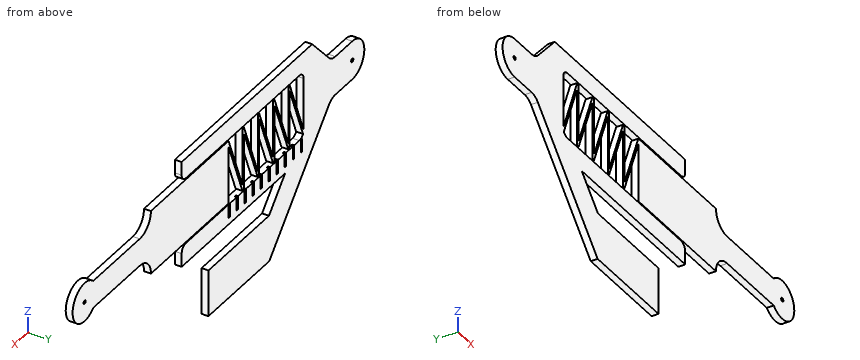
```python
from build123d import *

# Parameters (mm, degrees)
SKETCH3_R           = 0.8255
BOSS_EXTRUDE1_DEPTH = 3.175
SKETCH4_W           = 1
SKETCH4_H           = 6.35
CUT_EXTRUDE1_DEPTH  = 1


with BuildPart() as part:
    # Sketch3 → Boss-Extrude1 (new body)
    with BuildSketch(Plane(origin=(0, 0, 0), x_dir=(1, 0, 0), z_dir=(0, 1, 0))):
        with BuildLine():
            Line((-187.300108, 9), (-200.000108, 9))
            ThreePointArc((-200.000108, 9), (-209.000108, 0), (-200.000108, -9))
            Line((-200.000108, -9), (-187.300108, -9))
            ThreePointArc((-187.300108, -9), (-184.751148517, -9.534047322), (-182.630933912, -11.046360455))
            Line((-182.630933912, -11.046360455), (-170.000108, -24.75))
            Line((-170.000108, -24.75), (-72.500108, -24.75))
            Line((-72.500108, -24.75), (-72.500108, -18.525))
            ThreePointArc((-72.500108, -18.525), (-73.43004397, -16.27993597), (-75.675108, -15.35))
            Line((-75.675108, -15.35), (-160.475108, -15.35))
            ThreePointArc((-160.475108, -15.35), (-162.72017203, -14.42006403), (-163.650108, -12.175))
            Line((-163.650108, -12.175), (-163.650108, 12.175))
            Line((-163.650108, 12.175), (-153.250108, -14.85))
            Line((-153.250108, -14.85), (-152.250108, -14.85))
            Line((-152.250108, -14.85), (-152.250108, 12.090726648))
            Line((-152.250108, 12.090726648), (-141.820108, -14.732))
            Line((-141.820108, -14.732), (-140.820108, -14.732))
            Line((-140.820108, -14.732), (-140.820108, 12.090726648))
            Line((-140.820108, 12.090726648), (-130.390108, -14.732))
            Line((-130.390108, -14.732), (-129.390108, -14.732))
            Line((-129.390108, -14.732), (-129.390108, 12.090726648))
            Line((-129.390108, 12.090726648), (-118.960108, -14.732))
            Line((-118.960108, -14.732), (-117.960108, -14.732))
            Line((-117.960108, -14.732), (-117.960108, 12.090726648))
            Line((-117.960108, 12.090726648), (-107.530108, -14.732))
            Line((-107.530108, -14.732), (-49.530108, -14.732))
            ThreePointArc((-49.530108, -14.732), (-47.07507704, -8.80503096), (-41.148108, -6.35))
            Line((-41.148108, -6.35), (-6.377891501, -6.35))
            ThreePointArc((-6.377891501, -6.35), (9, 0), (-6.377891501, 6.35))
            Line((-6.377891501, 6.35), (-41.148108, 6.35))
            ThreePointArc((-41.148108, 6.35), (-47.07507704, 8.80503096), (-49.530108, 14.732))
            Line((-49.530108, 14.732), (-49.530108, 14.85))
            Line((-49.530108, 14.85), (-107.530108, 14.85))
            Line((-107.530108, 14.85), (-107.530108, -11.972726648))
            Line((-107.530108, -11.972726648), (-117.960108, 14.85))
            Line((-117.960108, 14.85), (-118.960108, 14.85))
            Line((-118.960108, 14.85), (-118.960108, -11.972726648))
            Line((-118.960108, -11.972726648), (-129.390108, 14.85))
            Line((-129.390108, 14.85), (-130.390108, 14.85))
            Line((-130.390108, 14.85), (-130.390108, -11.972726648))
            Line((-130.390108, -11.972726648), (-140.820108, 14.85))
            Line((-140.820108, 14.85), (-141.820108, 14.85))
            Line((-141.820108, 14.85), (-141.820108, -11.972726648))
            Line((-141.820108, -11.972726648), (-152.250108, 14.85))
            Line((-152.250108, 14.85), (-153.250108, 14.85))
            Line((-153.250108, 14.85), (-153.250108, -12.065668468))
            Line((-153.250108, -12.065668468), (-163.203485052, 13.798756035))
            ThreePointArc((-163.203485052, 13.798756035), (-162.044375279, 14.935077029), (-160.475108, 15.35))
            Line((-160.475108, 15.35), (-75.675108, 15.35))
            ThreePointArc((-75.675108, 15.35), (-73.43004397, 16.27993597), (-72.500108, 18.525))
            Line((-72.500108, 18.525), (-72.500108, 24.75))
            Line((-72.500108, 24.75), (-149.849684915, 24.75))
            Line((-149.849684915, 24.75), (-137.719938766, 37.91))
            Line((-137.719938766, 37.91), (-92.500108, 37.91))
            Line((-92.500108, 37.91), (-92.500108, 59.5))
            Line((-92.500108, 59.5), (-137.970573146, 59.5))
            Line((-137.970573146, 59.5), (-182.630933912, 11.046360455))
            ThreePointArc((-182.630933912, 11.046360455), (-184.751148517, 9.534047322), (-187.300108, 9))
        make_face()
        with Locations(Location((0, 0, 0), (0, 0, 270))):
            Circle(SKETCH3_R, mode=Mode.SUBTRACT)
        with Locations(Location((-200.000108, 0, 0), (0, 0, 270))):
            Circle(SKETCH3_R, mode=Mode.SUBTRACT)
    extrude(amount=BOSS_EXTRUDE1_DEPTH)

    # Sketch4 → Cut-Extrude1 (cut)
    with BuildSketch(Plane(origin=(0, 3.175, 0), x_dir=(1, 0, 0), z_dir=(0, 1, 0))):
        with Locations((-108.030108, 18.525)):
            Rectangle(SKETCH4_W, SKETCH4_H)
        with Locations((-114.030108, 18.525)):
            Rectangle(SKETCH4_W, SKETCH4_H)
        with Locations((-120.030108, 18.525)):
            Rectangle(SKETCH4_W, SKETCH4_H)
        with Locations((-126.030108, 18.525)):
            Rectangle(SKETCH4_W, SKETCH4_H)
        with Locations((-132.030108, 18.525)):
            Rectangle(SKETCH4_W, SKETCH4_H)
        with Locations((-138.030108, 18.525)):
            Rectangle(SKETCH4_W, SKETCH4_H)
        with Locations((-144.030108, 18.525)):
            Rectangle(SKETCH4_W, SKETCH4_H)
        with Locations((-150.030108, 18.525)):
            Rectangle(SKETCH4_W, SKETCH4_H)
        with Locations((-156.030108, 18.525)):
            Rectangle(SKETCH4_W, SKETCH4_H)
        with Locations((-162.030108, 18.525)):
            Rectangle(SKETCH4_W, SKETCH4_H)
    extrude(amount=-CUT_EXTRUDE1_DEPTH, mode=Mode.SUBTRACT)


solid = part.part
```
Source: CAD feature listing. Evaluate the final solid. Frame: model axes, mm. Coordinates: 2 decimals unless noted, no trailing zeros. Write each loop counter-clockwise with the first axis right and the second up, starting at its lowest first coordinate (ties: lowest second). Pieces come first, ordered by that corner, then holes. Notation, with made-up numbers: M 48,59 L 90,59 A20 cw 90,84 Z; hole C 73,80 d6. An arc over 180 degrees is marked long. Answer as a JSON object with one key per item and string values.
1. Ray query, L1, parallel to Z at x = -79.5, y = 1.05; L2, parallel to Y at x = -138.5, z = -17 (3 decimals); L3, parallel to X at y = 0.95, z = 14. Return the intervals inside material, ascending.
Evaluation:
{"L1": "-24.75 to -15.35, -14.85 to 14.73, 15.35 to 24.75", "L2": "0 to 2.175", "L3": "-179.91 to -163.07, -153.58 to -152.25, -142.1 to -140.82, -130.67 to -129.39, -119.24 to -117.96, -107.81 to -49.5"}
2. Contact query for flat-ended pins moving along their axis: P1, Ø0.8, axis at y = 3, z = -18.5, coming from the -X side; P2, Ø0.5, axis at y = 2.5, z = -17.5, coming from the -X side; P3, Ø1, axis at y = 2, z = -49.5, coming from the +X side. Output: stop coordinate, or through.
Evaluation:
{"P1": "x = -176.13", "P2": "x = -176.91", "P3": "x = -92.5"}
3. Cut plane B-B on y = 1.3. State how many separate pieces and enclosed holes the cut face has, plus the area to 3 significant figures.
Evaluation:
{"separate pieces": "1", "enclosed holes": "2", "area": "7,170 mm^2"}
4. Cut plane A-A on x = -80.5. Output: boundary loops of the cut face in (y, z) (3 decimals).
Evaluation:
{"outline": "M 0,-24.75 L 3.175,-24.75 L 3.175,-15.35 L 0,-15.35 Z; M 0,-14.85 L 3.175,-14.85 L 3.175,14.732 L 0,14.732 Z; M 0,15.35 L 3.175,15.35 L 3.175,24.75 L 0,24.75 Z"}
